```python
from build123d import *

# Parameters (mm, degrees)
PAD_DEPTH       = 2
SKETCH001_R     = 3
PAD001_DEPTH    = 2
SKETCH002_R     = 1.7
POCKET_DEPTH    = 5
SKETCH003_W     = 2
SKETCH003_H     = 36
PAD002_DEPTH    = 10
SKETCH004_R     = 22
POCKET001_DEPTH = 5


with BuildPart() as part:
    # Sketch → Pad (new body)
    with BuildSketch(Plane.XY):
        with BuildLine():
            Line((4.999993, 0), (115.000007, 0))
            ThreePointArc((115.000007, 0), (118.535542, 1.464474), (120, 5.000016))
            Line((120, 5.000016), (120, 54.999983))
            ThreePointArc((120, 54.999983), (118.535543, 58.535525), (115.000007, 60))
            Line((4.999993, 60), (115.000007, 60))
            ThreePointArc((4.999993, 60), (1.464457, 58.535525), (0, 54.999983))
            Line((0, 54.999983), (0, 5.000016))
            ThreePointArc((0, 5.000016), (1.464458, 1.464474), (4.999993, 0))
        make_face()
    extrude(amount=PAD_DEPTH)

    # Sketch001 → Pad001 (new body)
    with BuildSketch(Plane.XY.offset(2)):
        with Locations((20, 6)):
            Circle(SKETCH001_R)
        with Locations((71.9, 10.7)):
            Circle(SKETCH001_R)
        with Locations((71.9, 38.6)):
            Circle(SKETCH001_R)
        with Locations((21.1, 53.8)):
            Circle(SKETCH001_R)
    extrude(amount=PAD001_DEPTH)

    # Sketch002 → Pocket (cut)
    with BuildSketch(Plane.XY.offset(4)):
        with Locations((20, 6)):
            Circle(SKETCH002_R)
        with Locations((71.9, 10.7)):
            Circle(SKETCH002_R)
        with Locations((71.9, 38.6)):
            Circle(SKETCH002_R)
        with Locations((21.1, 53.8)):
            Circle(SKETCH002_R)
    extrude(amount=-POCKET_DEPTH, mode=Mode.SUBTRACT)

    # Sketch003 → Pad002 (new body)
    with BuildSketch(Plane.XY.offset(2)):
        with Locations((81, 30)):
            Rectangle(SKETCH003_W, SKETCH003_H)
    extrude(amount=PAD002_DEPTH)

    # Sketch004 → Pocket001 (cut)
    with BuildSketch(Plane.XY.offset(2)):
        with Locations((42, 30)):
            Circle(SKETCH004_R)
    extrude(amount=-POCKET001_DEPTH, mode=Mode.SUBTRACT)


solid = part.part
```
The model under review builds one solid part; all positions refer to its coordinate system, in mm. A direction names the side the tool comes from. Coordinates: 2 decimals unless noted, no trailing zeros. Write each loop counter-clockwise with the first axis right and the second up, starting at its lowest first coordinate (ties: lowest second). Pieces come first, ordered by that corner, then holes. Notation, with made-up numbers: (3.25, -4) -> (25.25, -4) arc R13 ccw to (25.25, 12) -> close; hole circle Ø3 at (52.5, 14.25). An arc over 180 degrees is marked (long way). One line per item, written item: value. Start each with the question number.
Q1. The part is to be moulded in two halves that separate along Y. For faces 4 (the face through (118, 1, 1)), 5 (the face through (73, 37, 4)), 6 (the face through (23.87, 52.65, 2.99)), say which applies: +Y half, -Y half, draft (parallel to the pull), parting line (faces both ways), or undercut.
Q2. Add section A-A, the plane x = 42. Give the boundary of the cut face in (y, z), then the cut area to 3 significant figures.
Q3. Add section B-B, the plane y = 53.8. Give the boundary of the cut face in (x, z).
Q4. To check wall thickness, follow probe 1 along Y at (x, z) = (71.9, 2.9); probe 2 along Y at (x, z) = (71.9, 1.9); probe 3 along X at (y, z) = (39, 10). State the ranges of each line that lie inside material, in increasing order.
Q5. Add section D-D, the plane z = 7. Give the boundary of the cut face in (x, y).
Q6. Clearance check with flat-ended pins moving along their axes: P1, Ø4, axis at x = 85.5, y = 26, coming from the +Z side; P2, Ø1.8, axis at x = 72, y = 11, coming from the +Z side; P3, Ø5, axis at x = 20.5, y = 7.5, coming from the +Z side; P4, Ø3, axis at y = 48, z = 5, coming from the +X side. State where each tip first meets the part, or that it passes through.
Q7. For faces 1 (the face through (82, 30, 7)), 2 (the face through (69.5, 36.8, 3)), 3 (the face through (73, 9, 4)), list the 3-axis set-ups (+Z, -Z, +X, -X, +Y, -Y) from which the entire face can be reached by the end or side of a thin tool; tool diameter is ignored.
Q8. Add section C-C, the plane y = 10.7. Give the boundary of the cut face in (x, z).
Response:
1. face 4: -Y half
1. face 5: draft
1. face 6: undercut
2. outline: (0, 0) -> (8, 0) -> (8, 2) -> (0, 2) -> close; (52, 0) -> (60, 0) -> (60, 2) -> (52, 2) -> close
2. area: 32.0 mm²
3. outline: (0, 0) -> (19.4, 0) -> (19.4, 4) -> (18.1, 4) -> (18.1, 2) -> (0, 2) -> close; (22.8, 0) -> (120, 0) -> (120, 2) -> (24.1, 2) -> (24.1, 4) -> (22.8, 4) -> close
4. probe 1: 7.7 to 9, 12.4 to 13.7, 35.6 to 36.9, 40.3 to 41.6
4. probe 2: 0 to 9, 12.4 to 36.9, 40.3 to 60
4. probe 3: 80 to 82
5. outline: (80, 12) -> (82, 12) -> (82, 48) -> (80, 48) -> close
6. P1: z = 2
6. P2: through
6. P3: z = 4
6. P4: x = 82
7. face 1: +Z, +X, +Y, -Y
7. face 2: +Z
7. face 3: +Z, -X, +Y, -Y
8. outline: (0, 0) -> (31.44, 0) -> (31.44, 2) -> (0, 2) -> close; (52.56, 0) -> (70.2, 0) -> (70.2, 4) -> (68.9, 4) -> (68.9, 2) -> (52.56, 2) -> close; (73.6, 0) -> (120, 0) -> (120, 2) -> (74.9, 2) -> (74.9, 4) -> (73.6, 4) -> close
